from build123d import *

# Parameters (mm, degrees)
SALIENTE_EXTRUIR1_DEPTH = 10
CROQUIS2_R              = 3.475
CORTAR_EXTRUIR1_DEPTH   = 21
CROQUIS3_R              = 4
SALIENTE_EXTRUIR2_DEPTH = 15
CROQUIS4_R              = 2.6
CORTAR_EXTRUIR2_DEPTH   = 6


with BuildPart() as part:
    # Croquis1 → Saliente-Extruir1 (new body, symmetric)
    with BuildSketch(Plane(origin=(0, 0, 0), x_dir=(1, 0, 0), z_dir=(0, 1, 0))):
        with BuildLine():
            Line((-59.5, 6.5), (0, 6.5))
            ThreePointArc((0, 6.5), (6.494269997, -0.272868487), (-0.545255886, -6.477090089))
            Line((-0.545255886, -6.477090089), (-59.835542084, -1.485901593))
            ThreePointArc((-59.835542084, -1.485901593), (-63.496473844, 2.667919069), (-59.5, 6.5))
        make_face()
    extrude(amount=SALIENTE_EXTRUIR1_DEPTH, both=True)

    # Croquis2 → Cortar-Extruir1 (cut, through all)
    with BuildSketch(Plane(origin=(0, 10, 0), x_dir=(1, 0, 0), z_dir=(0, 1, 0))):
        Circle(CROQUIS2_R)
    extrude(amount=-CORTAR_EXTRUIR1_DEPTH, mode=Mode.SUBTRACT)

    # Croquis3 → Saliente-Extruir2 (add)
    with BuildSketch(Plane(origin=(0, 10, 0), x_dir=(1, 0, 0), z_dir=(0, 1, 0))):
        with Locations((-59.5, 2.5)):
            Circle(CROQUIS3_R)
    extrude(amount=SALIENTE_EXTRUIR2_DEPTH)

    # Croquis4 → Cortar-Extruir2 (cut)
    with BuildSketch(Plane(origin=(0, 25, 0), x_dir=(1, 0, 0), z_dir=(0, 1, 0))):
        with Locations((-59.5, 2.5)):
            Circle(CROQUIS4_R)
    extrude(amount=-CORTAR_EXTRUIR2_DEPTH, mode=Mode.SUBTRACT)


solid = part.part
Input: part model. Units: mm. Frame: model coordinates. A direction names the side the tool comes from. Give positions to 0.01 mm unless a question says otherwise; leave off trailing zeros. Loops run counter-clockwise (first coordinate to the right, second up) from the corner with the lowest first, then second, coordinate; pieces in that order, holes last. Notation, with made-up numbers: M -1.75,33 L 19.25,33 A15 cw 19.25,61 Z; hole C 38.5,58.25 d4. An arc over 180 degrees is marked long. Use CSV: the item, a comma, the result in double quotes.
(1) Section C-C, the plane x = 1.5. Return loops of the section in (y, z), plus the area to 3 significant figures.
Outcome:
outline,"M -10,-6.32 L 10,-6.32 L 10,-3.13 L -10,-3.13 Z; M -10,3.13 L 10,3.13 L 10,6.32 L -10,6.32 Z"
area,"128 mm²"
(2) Section B-B, the plane z = -2.5. Return loops of the section in (x, y).
Outcome:
outline,"M -63.5,-10 L -2.41,-10 L -2.41,10 L -55.5,10 L -55.5,25 L -56.9,25 L -56.9,19 L -62.1,19 L -62.1,25 L -63.5,25 Z; M 2.41,-10 L 6,-10 L 6,10 L 2.41,10 Z"
(3) Pin query (flat end, axial travel): P1, Ø2, axis at x = -25, y = -1, coming from the +Z side; P2, Ø8, axis at x = -32, y = -3.5, coming from the +Z side; P3, Ø1, axis at x = -47.5, y = -5.5, coming from the +Z side. Return the tip coordinate at first contact, or that it passes through.
Outcome:
P1,"stops at z = 4.5"
P2,"stops at z = 4.17"
P3,"stops at z = 2.57"
(4) Material intervals for L1, parallel to Z at x = -59.5, y = 22.4; L2, parallel to Y at x = -22, z = -6; L3, parallel to Z at x = 0.5, y = -4, sorted ascending. Write a range as [from, to].
Outcome:
L1,"z = [-6.5, -5.1], [0.1, 1.5]"
L2,"y = [-10, 10]"
L3,"z = [-6.48, -3.44], [3.44, 6.48]"
(5) Set-up query: faces 1 (the face through (-62.1, 22, -2.6)), 2 (the face through (-56.9, 25, -3.4)). Return all of +Z, -Z, +X, -X, +Y, -Y with unobstructed straight access to the full face (end or side cutting, diameter ignored); none if empty.
Outcome:
face 1,"+Y"
face 2,"+Z, -Z, +X, -X, +Y"
(6) Section D-D, the plane y = -4. Return loops of the section in (x, z) (3 decimals), plus the area to 3 significant figures.
Outcome:
outline,"M -59.836,1.486 A4 ccw -59.5,-6.5 L 0,-6.5 A6.5 ccw long -0.545,6.477 Z; hole C 0,0 d6.95"
area,"679 mm²"
(7) Pull-direction query (Z, two-part tool) for faces 3 (the face through (6.5, 0.1, 0.1)), 4 (the face through (-60, 19, -3)), 5 (the face through (-26, 10, -2)); classes: pulls with the +Z half, pulls with the -Z half, needs draft (parallel to the pull), parting line crosses it, or undercut.
Outcome:
face 3,"parting line crosses it"
face 4,"undercut"
face 5,"needs draft"
(8) Section A-A, the plane y = 20. Return loops of the section in (x, z), plus the area to 3 significant figures.
Outcome:
outline,"C -59.5,-2.5 d8; hole C -59.5,-2.5 d5.2"
area,"29.0 mm²"
